Here's how the part is built. I have some questions about the finished solid (model axes, mm). A direction names the side the tool comes from. Give positions to 0.01 mm unless a question says otherwise; leave off trailing zeros. Loops run counter-clockwise (first coordinate to the right, second up) from the corner with the lowest first, then second, coordinate; pieces in that order, holes last. Notation, with made-up numbers: (-26.5, 66) - (26.5, 66) arc R25 cw to (26.5, 103) - close; hole circle Ø5 at (-6, 80). An arc over 180 degrees is marked (long way). Use a Markdown table: item, result.
from build123d import *

# Parameters (mm, degrees)
SKETCH2_R           = 5
CUT_EXTRUDE1_DEPTH  = 10
BOSS_EXTRUDE1_DEPTH = 0.5


with BuildPart() as part:
    # Sketch1 → Revolve1 (revolve)
    with BuildSketch(Plane.XY):
        Polygon((-13.622037679, 15.5), (0, 15.5), (0, 18), (2, 18), (2.8, 18), (2.8, 17.453091715), (2, 17.453091715), (2, 13.5), (-4.063478188, 13.5), (-5.311018839, 12.5), (-13.372037679, 12.5), (-14.622037679, 10.833333333), (-14.622037679, 0), (-16.622037679, 0), (-16.622037679, 11.5), align=None)
    revolve(axis=Axis((-25, 0, 0), (1, 0, 0)))

    # Sketch2 → Cut-Extrude1 (cut)
    with BuildSketch(Plane.ZY.offset(16.622037679)):
        Circle(SKETCH2_R)
    extrude(amount=-CUT_EXTRUDE1_DEPTH, mode=Mode.SUBTRACT)

    # Sketch3 → Boss-Extrude1 (add)
    with BuildSketch(Plane(origin=(-14.622037679, 0, 0), x_dir=(0, 0, -1), z_dir=(1, 0, 0))):
        Polygon((7.134838542, 3.062100229), (7.975608442, 3.633882224), (7.900815659, 4.647901314), (6.985252976, 5.090138409), (6.144483075, 4.518356414), (6.219275858, 3.504337324), align=None)
        Polygon((0.915562683, 7.710001544), (0.8407699, 8.724020633), (-0.074792783, 9.166257728), (-0.915562683, 8.594475733), (-0.8407699, 7.580456643), (0.074792783, 7.138219548), align=None)
        Polygon((6.219275858, -4.647901314), (7.134838542, -5.090138409), (7.975608442, -4.518356414), (7.900815659, -3.504337324), (6.985252976, -3.062100229), (6.144483075, -3.633882224), align=None)
        Polygon((-0.915562683, -7.710001544), (-0.8407699, -8.724020633), (0.074792783, -9.166257728), (0.915562683, -8.594475733), (0.8407699, -7.580456643), (-0.074792783, -7.138219548), align=None)
        Polygon((-7.134838542, -3.062100229), (-7.975608442, -3.633882224), (-7.900815659, -4.647901314), (-6.985252976, -5.090138409), (-6.144483075, -4.518356414), (-6.219275858, -3.504337324), align=None)
        Polygon((-6.219275858, 4.647901314), (-7.134838542, 5.090138409), (-7.975608442, 4.518356414), (-7.900815659, 3.504337324), (-6.985252976, 3.062100229), (-6.144483075, 3.633882224), align=None)
    extrude(amount=BOSS_EXTRUDE1_DEPTH)


solid = part.part
(1) Will these pins go through, and if not, where does the flat tip stop? pin 1 (8 mm diameter, centred on x = -6, z = 5.5, fed in from -Y); pin 2 (1.5 mm diameter, centred on y = -4.5, z = -7, fed in from +X); pin 3 (17.5 mm diameter, centred on y = -6, z = -3.5, fed in from +X); pin 4 (8 mm diameter, centred on y = 0, z = 0, fed in from +X).
A:
| item | result |
|---|---|
| pin 1 | y = -15.43 |
| pin 2 | x = -14.12 |
| pin 3 | x = 2 |
| pin 4 | through |
(2) Suppose I cut it at C-C on x = -3. Write out the boundary of the cut face in (y, z).
A:
| item | result |
|---|---|
| outline | circle Ø31 at (0, 0); hole circle Ø27 at (0, 0) |
(3) Suppose I cut it at B-B on x = -9.75. Write out the boundary of the cut face in (y, z), plus the area to 3 significant figures.
A:
| item | result |
|---|---|
| outline | circle Ø31 at (0, 0); hole circle Ø25 at (0, 0) |
| area | 264 mm2 |
(4) Suppose I cut it at A-A on y = 0. Write out the boundary of the cut face in (x, z), plus the area to 3 significant figures.
A:
| item | result |
|---|---|
| outline | (-16.62, -11.5) - (-13.62, -15.5) - (0, -15.5) - (0, -18) - (2.8, -18) - (2.8, -17.45) - (2, -17.45) - (2, -13.5) - (-4.06, -13.5) - (-5.31, -12.5) - (-13.37, -12.5) - (-14.62, -10.83) - (-14.62, -5) - (-16.62, -5) - close; (-16.62, 5) - (-14.62, 5) - (-14.62, 10.83) - (-13.37, 12.5) - (-5.31, 12.5) - (-4.06, 13.5) - (2, 13.5) - (2, 17.45) - (2.8, 17.45) - (2.8, 18) - (0, 18) - (0, 15.5) - (-13.62, 15.5) - (-16.62, 11.5) - close |
| area | 129 mm2 |
(5) If I drill on line 1 (Z direction, x = -0.5, y = 0); line 2 (X direction, y = 12, z = -7.5); line 3 (Z direction, x = 1.5, y = -8), over which ranges is the centre line in solid material (lowest first)?
A:
| item | result |
|---|---|
| line 1 | -15.5 to -13.5, 13.5 to 15.5 |
| line 2 | -14.63 to 2 |
| line 3 | -16.12 to -10.87, 10.87 to 16.12 |
(6) On a 3-axis mill with a long thin cutter (end or side, diameter ignored), from which of +Z, -Z, +X, -X, +Y, -Y can I reach the whole of each face in a straight line? I mean faces 1 (the face through (-16.622, -5, -2)), 2 (the face through (-6.716, -2.018, 15.368)), 3 (the face through (-14.122, -4, 7)). Say none if no direction works.
A:
| item | result |
|---|---|
| face 1 | +Z, -Z, -X, +Y, -Y |
| face 2 | -X |
| face 3 | +X |
(7) We'd pull the mould along Y, two halves only. Please class faces 4 (the face through (-14.122, 4, -7)), 5 (the face through (-16.434, 11.208, 3.529)), 6 (the face through (2.8, -2.8, 17.4)): pulls with the +Y half, pulls with the -Y half, needs draft (parallel to the pull), parting line crosses it, or undercut.
A:
| item | result |
|---|---|
| face 4 | undercut |
| face 5 | parting line crosses it |
| face 6 | needs draft |
